Could you check a few things on this model? Use its own coordinates, in mm. Face numbers are marked on the shaded views. A direction names the side the tool comes from. Give positions to 0.01 mm unless a question says otherwise; leave off trailing zeros. Order: outer loops, then holes, each group sorted by start corner. A loop starts at its lowest first (then second) coordinate and runs counter-clockwise, first axis right, second up. Notation, with made-up numbers: (-36.5, 8.25) -> (-1.5, 8.25) arc R25 cw to (-1.5, 30.25) -> close; hole circle Ø10 at (50.5, 77). An arc over 180 degrees is marked (long way). One line per item, written item: value.
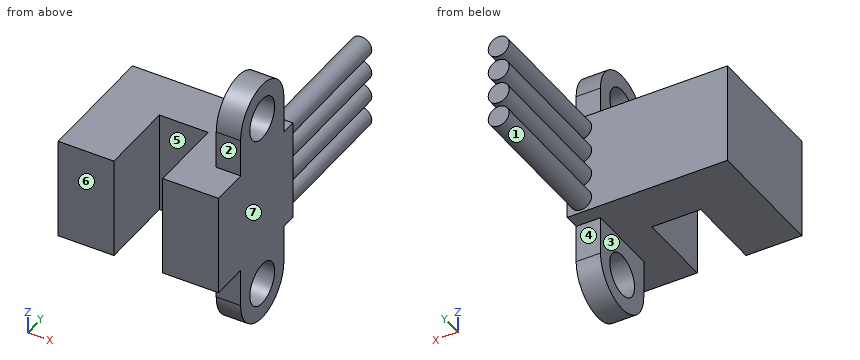
```python
from build123d import *

# Parameters (mm, degrees)
BOSS_EXTRU_1_DEPTH = 3.65
ESQUISSE2_R        = 1.5
BOSS_EXTRU_2_DEPTH = 1.75
ESQUISSE3_R        = 0.75
BOSS_EXTRU_3_DEPTH = 10


with BuildPart() as part:
    # Esquisse1 → Boss.-Extru.1 (new, symmetric)
    with BuildSketch(Plane.XY):
        Polygon((1.75, 0), (-1.75, 0), (-1.75, -5.5), (-5.75, -5.5), (-5.75, 3.5), (5.75, 3.5), (5.75, -5.5), (1.75, -5.5), align=None)
    extrude(amount=BOSS_EXTRU_1_DEPTH, both=True)

    # Esquisse2 → Boss.-Extru.2 (add)
    with BuildSketch(Plane(origin=(5.75, 0, 0), x_dir=(0, 0, -1), z_dir=(1, 0, 0))):
        with BuildLine():
            Line((-6.375, 2.42), (-3.65, 2.42))
            Line((-3.65, 2.42), (-3.65, -2.82))
            Line((-3.65, -2.82), (-6.375, -2.82))
            ThreePointArc((-6.375, -2.82), (-8.995, -0.2), (-6.375, 2.42))
        make_face()
        with Locations((-6.375, -0.2)):
            Circle(ESQUISSE2_R, mode=Mode.SUBTRACT)
    boss_extru_2 = extrude(amount=-BOSS_EXTRU_2_DEPTH)

    # Symétrie1: Boss.-Extru.2 across plane
    add(boss_extru_2.mirror(Plane.XY))

    # Esquisse3 → Boss.-Extru.3 (add)
    with BuildSketch(Plane(origin=(0, 3.5, 0), x_dir=(1, 0, 0), z_dir=(0, 1, 0))):
        with Locations((4.75, 2.7)):
            Circle(ESQUISSE3_R)
        with Locations((4.75, 0.9)):
            Circle(ESQUISSE3_R)
        with Locations((4.75, -0.9)):
            Circle(ESQUISSE3_R)
        with Locations((4.75, -2.7)):
            Circle(ESQUISSE3_R)
    extrude(amount=BOSS_EXTRU_3_DEPTH)


solid = part.part
```
1) Suppose I cut it at D-D, the plane z = -7. Write out the boundary of the cut face in (x, y).
Answer below:
outline: (4, -2.74) -> (5.75, -2.74) -> (5.75, -1.56) -> (4, -1.56) -> close; (4, 1.16) -> (5.75, 1.16) -> (5.75, 2.34) -> (4, 2.34) -> close
2) Suppose I cut it at C-C, the plane y = -3.5. Write out the boundary of the cut face in (x, z), then the cut area to 3 significant figures.
Answer below:
outline: (-5.75, -3.65) -> (-1.75, -3.65) -> (-1.75, 3.65) -> (-5.75, 3.65) -> close; (1.75, -3.65) -> (5.75, -3.65) -> (5.75, 3.65) -> (1.75, 3.65) -> close
area: 58.4 mm2
3) For the marked faces 1, 2, 3 and 4, which set-ups out of +Z, -Z, +X, -X, +Y, -Y let a thin tool reach every point of the face, with its end or its side?
Answer below:
face 1: +Y
face 2: +Z, +X, -X, -Y
face 3: -Z, -X, +Y, -Y
face 4: -Z, +X, -X, +Y
4) If I drill on line 1 along Z through (x, y) = (4.5, 0.5); line 2 along X through (y, z) = (-1.5, 0.75); line 3 along Y through (x, z) = (2, -1.75), over which ranges is the centre line in solid material (lowest first)?
Answer below:
line 1: z = -8.9 to -7.7, -5.05 to 5.05, 7.7 to 8.9
line 2: x = -5.75 to -1.75, 1.75 to 5.75
line 3: y = -5.5 to 3.5
5) We'd pull the mould along X, two halves only. Please class the marked faces 5, 6 and 7: +X half, -X half, draft (parallel to the pull), parting line (faces both ways), or undercut.
Answer below:
face 5: undercut
face 6: draft
face 7: +X half
6) For P1, Ø0.9, axis at x = 4.5, z = 5.5, coming from the +Y side; P2, Ø6, axis at y = 0.5, z = -5.5, coming from the -X side; P3, Ø2.5, axis at y = -0.2, z = 6.375, coming from the +X side; P4, Ø8, axis at y = 11.5, z = -1.5, coming from the +X side, each with a flat end and sliding along its axis, tell me the tip position at first contact or that it passes through.
Answer below:
P1: stops at y = 2.42
P2: stops at x = -5.75
P3: passes through
P4: stops at x = 5.5
7) Suppose I cut it at A-A, the plane x = 4.75. State how many separate pieces and enclosed holes the cut face has, then the cut area to 3 significant figures.
Answer below:
separate pieces: 1
enclosed holes: 2
area: 162 mm2
8) Suppose I cut it at B-B, the plane z = 2.25. Write out the boundary of the cut face in (x, y).
Answer below:
outline: (-5.75, -5.5) -> (-1.75, -5.5) -> (-1.75, 0) -> (1.75, 0) -> (1.75, -5.5) -> (5.75, -5.5) -> (5.75, 3.5) -> (5.35, 3.5) -> (5.35, 13.5) -> (4.15, 13.5) -> (4.15, 3.5) -> (-5.75, 3.5) -> close
